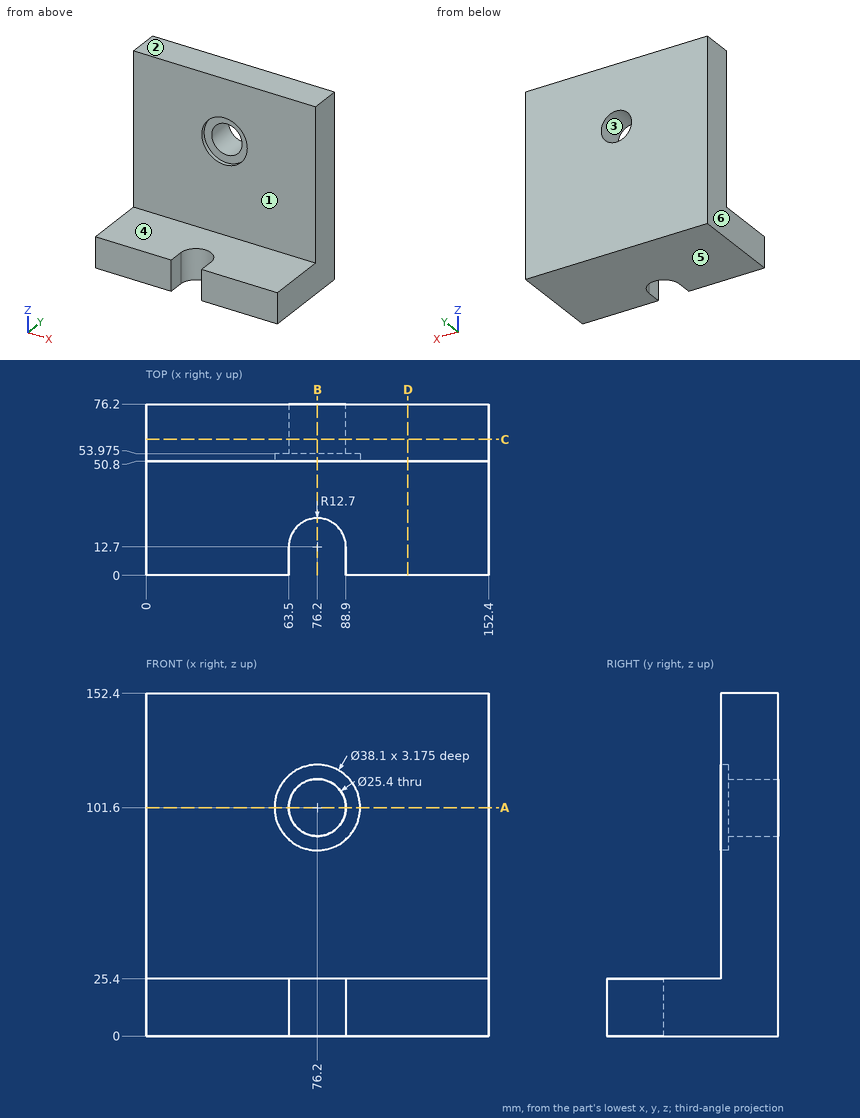
Print and shaded views of the part. All mm, measured from the part's lowest x, y and z. A direction names the side the tool comes from. Round coordinates to 2 decimals unless told otherwise and drop trailing zeros. Write each loop counter-clockwise with the first axis right and the second up, starting at its lowest first coordinate (ties: lowest second). Pieces come first, ordered by that corner, then holes.
(1) Slice it at C-C, the plane y = 60.5. Write the cut outline in (x, z), and give its area (3 significant figures).
(2) Slice it at A-A, the plane z = 101.6. Write the cut outline in (x, y) (3 decimals), and give its area (3 significant figures).
(3) Slice it at B-B, the plane x = 76.2. Write the cut outline in (y, z) (3 decimals).
(4) Slice it at D-D, the plane x = 116.5. Write the cut outline in (y, z), and give its area (3 significant figures).
(5) Probe line 1 along X through (y, z) = (62, 101.6); line 2 along Z through (x, y) = (76, 70); line 3 along Z through (x, y) = (105, 26). List the from-to ranges inside material, lowest first.
(6) 3-axis set-ups, long thin cutter, end or side, ignore diameter. For the marked faces 1 and 2: which of +Z, -Z, +X, -X, +Y, -Y reach the whole face in a straight line?
(7) Drop flat-ended pins along their axis: P1, Ø6, axis at x = 105, z = 132.5, coming from the -Y side; P2, Ø20.5, axis at x = 76.2, z = 101.6, coming from the -Y side. Give the stop position or say it passes through.
(8) Mould opens along Z. For the marked faces 3, 4, 5 and 6 say: pulls with the +Z half, pulls with the -Z half, needs draft (parallel to the pull), parting line crosses it, or undercut.
From the geometry:
1. outline: (0, 0) - (152.4, 0) - (152.4, 152.4) - (0, 152.4) - close; hole circle Ø25.4 at (76.2, 101.6)
1. area: 22,700 mm2
2. outline: (0, 50.8) - (57.15, 50.8) - (57.15, 53.975) - (63.5, 53.975) - (63.5, 76.2) - (0, 76.2) - close; (88.9, 53.975) - (95.25, 53.975) - (95.25, 50.8) - (152.4, 50.8) - (152.4, 76.2) - (88.9, 76.2) - close
2. area: 3,190 mm2
3. outline: (25.4, 0) - (76.2, 0) - (76.2, 88.9) - (53.975, 88.9) - (53.975, 82.55) - (50.8, 82.55) - (50.8, 25.4) - (25.4, 25.4) - close; (50.8, 120.65) - (53.975, 120.65) - (53.975, 114.3) - (76.2, 114.3) - (76.2, 152.4) - (50.8, 152.4) - close
4. outline: (0, 0) - (76.2, 0) - (76.2, 152.4) - (50.8, 152.4) - (50.8, 25.4) - (0, 25.4) - close
4. area: 5,160 mm2
5. line 1: x = 0 to 63.5, 88.9 to 152.4
5. line 2: z = 0 to 88.9, 114.3 to 152.4
5. line 3: z = 0 to 25.4
6. face 1: +Z, +X, -X, -Y
6. face 2: +Z, +X, -X, +Y, -Y
7. P1: stops at y = 50.8
7. P2: passes through
8. face 3: undercut
8. face 4: pulls with the +Z half
8. face 5: pulls with the -Z half
8. face 6: needs draft
